CAD build for the part. Positions are in the model's coordinates, mm. A direction names the side the tool comes from. Round coordinates to 2 decimals unless told otherwise and drop trailing zeros. Write each loop counter-clockwise with the first axis right and the second up, starting at its lowest first coordinate (ties: lowest second). Pieces come first, ordered by that corner, then holes. Notation, with made-up numbers: (53, 44) - (63, 44) arc R31 ccw to (63, 79) - close; hole circle Ø7 at (86.25, 59.5). An arc over 180 degrees is marked (long way). Put each result on its own line as item: value. Start each with the question number.
Item 1: Cut at A-A (y = 264). Give the cut face in (x, z).
Item 2: Mould opens along Z. For faces 4 (the flat face through (-467.85, 249.678, -49.638)), 5 (the flat face through (-456, 266, -25.4)), 6 (the flat face through (-460, 265, 3.81)), 7 (the flat face through (-470.818, 265, -12)) say: released by +Z, released by -Z, zero draft, split by the parting line, or undercut.
Item 3: Cut at B-B (z = -8.5). Give the cut face in (x, y), and give its area (3 significant figures).
Item 4: Drill centre lines: line 1 (Y direction, x = -463, z = -0.5); line 2 (Z direction, x = -456, y = 265); line 3 (Y direction, x = -458.5, z = 1.5). Where is each one in solid material? Low to high. Write a range as from..to.
Item 5: Pin check, flat tips, straight feed: pin 1 Ø8.5 at (x, y) = (-456, 271.99) entering from -Z; pin 2 Ø6 at (x, y) = (-469, 252) entering from -Z; pin 3 Ø2 at (x, y) = (-474.5, 248) entering from -Z; pin 4 Ø5 at (y, z) = (273, -30) entering from +X. Stop position of each tip, or through.
Item 6: 3-axis set-ups, long thin cutter, end or side, ignore diameter. For faces 1 (the flat face through (-453.98, 253.72, -12.52)), 2 (the flat face through (-456, 266, 0)), 3 (the cylindrical face through (-464.55, 249.23, -41.17)): which of +Z, -Z, +X, -X, +Y, -Y reach the whole face in a straight line?
Item 7: Cut at D-D (z = -20). Give the cut face in (x, y).
Item 8: Cut at C-C (x = -455.75). Give the cut face in (y, z).
```python
from build123d import *

# Parameters (mm, degrees)
BOSS_EXTRUDE1_DEPTH = 27.94
SKETCH2_W           = 21.59
SKETCH2_H           = 28.064626237
SKETCH2_R           = 3.175
BOSS_EXTRUDE2_DEPTH = 3.81
SKETCH3_R           = 3.175
BOSS_EXTRUDE3_DEPTH = 2.54
SKETCH4_W           = 21.59
SKETCH4_H           = 73.66
SKETCH4_R           = 3.175
BOSS_EXTRUDE4_DEPTH = 5.588
BOSS_EXTRUDE5_DEPTH = 21.59


with BuildPart() as part:
    # Sketch1 → Boss-Extrude1 (new body)
    with BuildSketch(Plane.XY):
        with BuildLine():
            ThreePointArc((-461.366897066, 277.506071532), (-460.543620658, 278.201967285), (-459.631228606, 278.776071532))
            Line((-459.631228606, 278.776071532), (-470.817858916, 278.776071532))
            Line((-470.817858916, 278.776071532), (-470.817858916, 250.711445295))
            Line((-470.817858916, 250.711445295), (-449.227858916, 250.711445295))
            Line((-449.227858916, 250.711445295), (-449.227858916, 252.940469765))
            Line((-449.227858916, 252.940469765), (-458.862647092, 254.521445295))
            ThreePointArc((-458.862647092, 254.521445295), (-461.281801172, 255.348530126), (-463.296789086, 256.922124572))
            ThreePointArc((-463.296789086, 256.922124572), (-463.938709782, 257.725469547), (-464.467858916, 258.607187485))
            ThreePointArc((-464.467858916, 258.607187485), (-465.307742726, 262.469481888), (-464.120754615, 266.239598875))
            ThreePointArc((-464.120754615, 266.239598875), (-463.399405765, 268.135304283), (-463.477224231, 270.162121354))
            ThreePointArc((-463.477224231, 270.162121354), (-463.397272377, 274.114329254), (-461.366897066, 277.506071532))
        make_face()
    extrude(amount=-BOSS_EXTRUDE1_DEPTH)

    # Sketch2 → Boss-Extrude2 (add)
    with BuildSketch(Plane.XY):
        with Locations((-460.022858916, 264.743758414)):
            Rectangle(SKETCH2_W, SKETCH2_H)
        with Locations(Location((-455.996603091, 271.987703521, 0), (0, 0, 180))):
            Circle(SKETCH2_R, mode=Mode.SUBTRACT)
        with Locations(Location((-457.615851502, 262.119672583, 0), (0, 0, 180))):
            Circle(SKETCH2_R, mode=Mode.SUBTRACT)
    extrude(amount=BOSS_EXTRUDE2_DEPTH)

    # Sketch3 → Boss-Extrude3 (add)
    with BuildSketch(Plane(origin=(0, 0, -25.4), x_dir=(-1, 0, 0), z_dir=(0, 0, -1))):
        with BuildLine():
            Line((449.227858916, 252.940469765), (449.227858916, 278.776071532))
            Line((449.227858916, 278.776071532), (459.631228606, 278.776071532))
            ThreePointArc((459.631228606, 278.776071532), (463.027763128, 275.12700781), (463.477224231, 270.162121354))
            ThreePointArc((463.477224231, 270.162121354), (463.399405765, 268.135304283), (464.120754615, 266.239598875))
            ThreePointArc((464.120754615, 266.239598875), (464.640877411, 258.967440337), (458.862647092, 254.521445295))
            Line((458.862647092, 254.521445295), (449.227858916, 252.940469765))
        make_face()
        with Locations((455.996603091, 271.987703521)):
            Circle(SKETCH3_R, mode=Mode.SUBTRACT)
        with Locations((457.615851502, 262.119672583)):
            Circle(SKETCH3_R, mode=Mode.SUBTRACT)
    extrude(amount=BOSS_EXTRUDE3_DEPTH)

    # Sketch4 → Boss-Extrude4 (add)
    with BuildSketch(Plane(origin=(3.845560936, 242.063082319, 11.417237821), x_dir=(0.9998741117550617, -0.01584934704377417, -0.0007475562269394038), z_dir=(0.01586696700779418, 0.9987637706378838, 0.04710806533037051))):
        with Locations((-471.560049375, 24.516249071)):
            Rectangle(SKETCH4_W, SKETCH4_H)
        with Locations(Location((-471.560049375, 52.456249071, 0), (0, 0, 270))):
            Circle(SKETCH4_R, mode=Mode.SUBTRACT)
        with Locations(Location((-471.560049375, -3.423750929, 0), (0, 0, 270))):
            Circle(SKETCH4_R, mode=Mode.SUBTRACT)
    extrude(amount=-BOSS_EXTRUDE4_DEPTH)

    # Sketch5 → Boss-Extrude5 (add)
    with BuildSketch(Plane.ZY.offset(470.817858916)):
        Polygon((3.81, 250.711445295), (3.81, 250.083908323), (-13.668693003, 250.908314891), align=None)
    extrude(amount=-BOSS_EXTRUDE5_DEPTH)


solid = part.part
```
Output values:
1. outline: (-470.82, -27.94) - (-460.17, -27.94) - (-460.17, -25.4) - (-465.08, -25.4) - (-465.08, 0) - (-460.17, 0) - (-460.17, 3.81) - (-470.82, 3.81) - close; (-455.06, -27.94) - (-449.23, -27.94) - (-449.23, -25.4) - (-455.06, -25.4) - close; (-455.06, 0) - (-449.23, 0) - (-449.23, 3.81) - (-455.06, 3.81) - close
2. face 4: released by -Z
2. face 5: undercut
2. face 6: released by +Z
2. face 7: zero draft
3. outline: (-478.54, 245.07) - (-456.95, 244.73) - (-456.86, 250.32) - (-478.45, 250.66) - close; (-470.82, 250.66) - (-449.23, 250.66) - (-449.23, 252.94) - (-458.86, 254.52) arc R7.7 cw to (-464.12, 266.24) arc R5.08 ccw to (-463.48, 270.16) arc R7.7 cw to (-459.63, 278.78) - (-470.82, 278.78) - close
3. area: 373 mm2
4. line 1: 244.45..250.04, 250.29..256.62, 275.19..278.78
4. line 2: -27.94..-25.4, 0..3.81
4. line 3: 244.28..249.88, 250.19..259.07, 265.17..270.03, 273.94..278.78
5. pin 1: z = -27.94
5. pin 2: z = -49.67
5. pin 3: z = -49.76
5. pin 4: x = -449.23
6. face 1: +X, +Y
6. face 2: +X
6. face 3: none
7. outline: (-478.54, 245.61) - (-456.95, 245.27) - (-456.86, 250.71) - (-449.23, 250.71) - (-449.23, 252.94) - (-458.86, 254.52) arc R7.7 cw to (-464.12, 266.24) arc R5.08 ccw to (-463.48, 270.16) arc R7.7 cw to (-459.63, 278.78) - (-470.82, 278.78) - (-470.82, 251.09) - (-478.45, 251.21) - close
8. outline: (250.08, 3.81) - (250.71, -9.49) - (250.71, -27.94) - (259.55, -27.94) - (259.55, -25.4) - (254.01, -25.4) - (254.01, 0) - (259.55, 0) - (259.55, 3.81) - close; (264.69, -27.94) - (268.82, -27.94) - (268.82, -25.4) - (264.69, -25.4) - close; (264.69, 0) - (268.82, 0) - (268.82, 3.81) - (264.69, 3.81) - close; (275.15, -27.94) - (278.78, -27.94) - (278.78, -25.4) - (275.15, -25.4) - close; (275.15, 0) - (278.78, 0) - (278.78, 3.81) - (275.15, 3.81) - close
